CAD build for the part. Positions are in the model's coordinates, mm. Round coordinates to 2 decimals unless told otherwise and drop trailing zeros. Loops run counter-clockwise (first coordinate to the right, second up) from the corner with the lowest first, then second, coordinate; pieces in that order, holes last. Notation, with made-up numbers: M -23.75,-6 L 19.25,-6 A27 cw 19.25,18 Z; hole C 66,-21 d1. An arc over 180 degrees is marked long. Use a Markdown table: item, result. Add a question column.
(1) Flat gauge pin, fed straight in: P1, Ø2, axis at x = 24.5, z = 1, coming from the +Y side. Where does the tip first touch, or does it go through?
(2) Band-saw the part on A-A, the plane z = 3.2. Write the cut outline in (x, y), and give its area (3 significant figures).
(3) Band-saw the part on B-B, the plane x = -18. Write the cut outline in (y, z).
(4) Wall check: L1, parallel to Y at x = -32.5, z = 2.15. Give the ranges that are in metal, low to high.
Autodesk Inventor part; units mm, degrees
ref_plane "YZ Plane" through (0, 0, 0) normal (1, 0, 0) x (0, 1, 0)
ref_plane "XZ Plane" through (0, 0, 0) normal (0, 1, 0) x (-1, 0, 0)
ref_plane "XY Plane" through (0, 0, 0) normal (0, 0, 1) x (1, 0, 0)
sketch "Sketch1" plane through (0, 0, 0) normal (0, 0, 1) x (1, 0, 0)
  line L0 (65, -70) -> (65, 70)
  line L1 (-65, 70) -> (-65, -70)
  line L2 (-65, 70) -> (-65, 65)
  line L3 (-15, 65) -> (-15, 70)
  line L4 (-15, 65) -> (-35, 65)
  line L5 (-35, 65) -> (-35, 70)
  line L6 (15, 65) -> (15, 70)
  line L7 (35, 65) -> (35, 70)
  line L8 (-35, 70) -> (-65, 70)
  line L9 (65, 70) -> (35, 70)
  line L10 (15, 70) -> (-15, 70)
  line L11 (-15, -65) -> (-15, -70)
  line L12 (-15, -65) -> (-35, -65)
  line L13 (-35, -65) -> (-35, -70)
  line L14 (35, -65) -> (35, -70)
  line L15 (15, -65) -> (15, -70)
  line L16 (-35, -70) -> (-65, -70)
  line L17 (65, -70) -> (35, -70)
  line L18 (15, -70) -> (-15, -70)
  line L19 (-65, -70) -> (-35, -70)
  line L20 (35, -70) -> (65, -70)
  line L21 (-35, -65) -> (-15, -65)
  line L22 (15, -65) -> (35, -65)
  line L23 (-35, 65) -> (-15, 65)
  line L24 (15, 65) -> (35, 65)
  point P0 (0, 0)
extrude "Extrusion1" add sketch "Sketch1" along normal blind 4
sketch "Sketch2" plane through (-15, 70, 0) normal (0, 1, 0) x (1, 0, 0)
  line L0 (-20, 0) -> (-50, 0)
  line L1 (-50, 0) -> (-50, -4)
  line L2 (-20, -4) -> (-50, -4)
  line L3 (-20, 0) -> (-20, -4)
  line L4 (0, 0) -> (-20, 0)
  line L5 (-20, 0) -> (-20, -4)
  line L6 (0, -4) -> (-20, -4)
  line L7 (0, 0) -> (0, -4)
  line L8 (30, 0) -> (0, 0)
  line L9 (0, 0) -> (0, -4)
  line L10 (30, -4) -> (0, -4)
  line L11 (30, 0) -> (30, -4)
  line L12 (50, 0) -> (30, 0)
  line L13 (50, -4) -> (30, -4)
  line L14 (50, 0) -> (30, 0)
  line L15 (30, 0) -> (30, -4)
  line L16 (50, -4) -> (30, -4)
  line L17 (50, 0) -> (50, -4)
  line L18 (80, 0) -> (50, 0)
  line L19 (50, 0) -> (50, -4)
  line L20 (80, -4) -> (50, -4)
  line L21 (80, 0) -> (80, -4)
  point P0 (15, 0)
properties part number "torso_base"
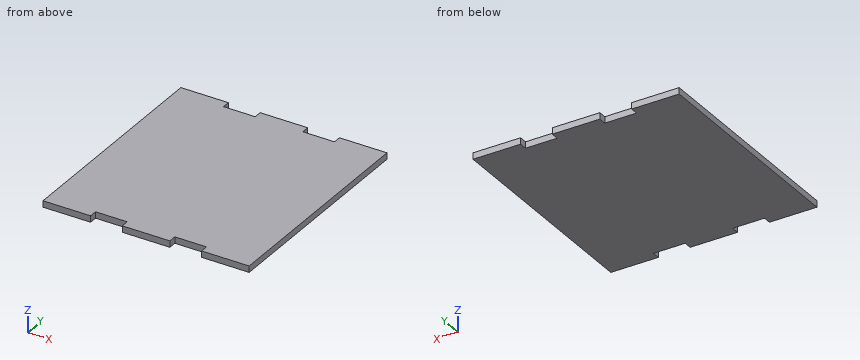
Return value:
| question | item | result |
|---|---|---|
| 1 | P1 | y = 65 |
| 2 | outline | M -65,-70 L -35,-70 L -35,-65 L -15,-65 L -15,-70 L 15,-70 L 15,-65 L 35,-65 L 35,-70 L 65,-70 L 65,70 L 35,70 L 35,65 L 15,65 L 15,70 L -15,70 L -15,65 L -35,65 L -35,70 L -65,70 Z |
| 2 | area | 17,800 mm^2 |
| 3 | outline | M -65,0 L 65,0 L 65,4 L -65,4 Z |
| 4 | L1 | -65 to 65 |
